```python
from build123d import *

# Parameters (mm, degrees)
MODEL_R             = 1.3
MODEL_R_2           = 1.344067797
MODEL_W             = 12.2
MODEL_H             = 22.8
BOSS_EXTRUDE1_DEPTH = 3


with BuildPart() as part:
    # Model → Boss-Extrude1 (new body)
    with BuildSketch(Plane.XY):
        with BuildLine():
            Line((25.639766947, 69.089607729), (69.59281779, 69.089607729))
            ThreePointArc((69.59281779, 69.089607729), (71.883249375, 68.155605213), (72.834203695, 65.872159696))
            Line((72.834203695, 65.872159696), (72.834203695, 21.872118121))
            ThreePointArc((72.834203695, 21.872118121), (71.882847983, 19.587552286), (69.590964861, 18.653962174))
            Line((69.590964861, 18.653962174), (25.641619876, 18.653962174))
            ThreePointArc((25.641619876, 18.653962174), (23.349724106, 19.587556709), (22.398372881, 21.872138909))
            Line((22.398372881, 21.872138909), (22.398372881, 65.872138909))
            ThreePointArc((22.398372881, 65.872138909), (23.349322718, 68.155600786), (25.639766947, 69.089607729))
        make_face()
        with Locations((25.616288319, 65.871777925)):
            Circle(MODEL_R, mode=Mode.SUBTRACT)
        with Locations((69.616288319, 65.871777925)):
            Circle(MODEL_R, mode=Mode.SUBTRACT)
        with Locations((56.616292368, 43.872138909)):
            Circle(MODEL_R_2, mode=Mode.SUBTRACT)
        with Locations((38.616292368, 43.872138909)):
            Circle(MODEL_R_2, mode=Mode.SUBTRACT)
        with Locations((25.616288319, 21.871777925)):
            Circle(MODEL_R, mode=Mode.SUBTRACT)
        with Locations((69.616288319, 21.871777925)):
            Circle(MODEL_R, mode=Mode.SUBTRACT)
        with Locations((47.616292368, 43.872138909)):
            Rectangle(MODEL_W, MODEL_H, mode=Mode.SUBTRACT)
    extrude(amount=BOSS_EXTRUDE1_DEPTH)


solid = part.part
```
The listing builds one solid part. Answer for the finished solid, in the listing's coordinates (mm). A direction names the side the tool comes from. Give positions to 0.01 mm unless a question says otherwise; leave off trailing zeros. Order: outer loops, then holes, each group sorted by start corner. A loop starts at its lowest first (then second) coordinate and runs counter-clockwise, first axis right, second up.
Item 1: Find the intervals of material crossed by probe 1 along X at (y, z) = (66, 1.3); probe 2 along X at (y, z) = (33, 0.75); probe 3 along Y at (x, z) = (70.5, 1.7), in increasing order.
From the geometry:
probe 1: x = 22.4 to 24.32, 26.91 to 68.32, 70.91 to 72.83
probe 2: x = 22.4 to 41.52, 53.72 to 72.83
probe 3: y = 18.78 to 20.92, 22.83 to 64.92, 66.83 to 68.97
Item 2: The part is cut by section B-B, the plane z = 0.6. Give the vertices of the cut face in (x, y).
From the geometry:
outline: (22.4, 21.87) arc R3.22 ccw to (25.64, 18.65) - (69.59, 18.65) arc R3.22 ccw to (72.83, 21.87) - (72.83, 65.87) arc R3.22 ccw to (69.59, 69.09) - (25.64, 69.09) arc R3.22 ccw to (22.4, 65.87) - close; hole circle Ø2.6 at (25.62, 21.87); hole circle Ø2.6 at (25.62, 65.87); hole circle Ø2.69 at (38.62, 43.87); hole (41.52, 32.47) - (53.72, 32.47) - (53.72, 55.27) - (41.52, 55.27) - close; hole circle Ø2.69 at (56.62, 43.87); hole circle Ø2.6 at (69.62, 21.87); hole circle Ø2.6 at (69.62, 65.87)
Item 3: For a pull along Y with two mould halves and no side action, classify faces 1 (the face through (72.834, 44, 1)), 2 (the face through (53.716, 44, 1)), 3 (the face through (23.324, 68.13, 1.479)) as pulls with the +Y half, pulls with the -Y half, needs draft (parallel to the pull), parting line crosses it, or undercut.
From the geometry:
face 1: needs draft
face 2: undercut
face 3: pulls with the +Y half
Item 4: Which of the six approach directions +Z, -Z, +X, -X, +Y, -Y give full straight-line access (tool end or side, diameter ignored) to faces 4 (the face through (48, 55.272, 1)), 5 (the face through (47.97, 55.43, 0))?
From the geometry:
face 4: +Z, -Z
face 5: -Z, +X, -X, +Y, -Y
Item 5: The part is cut by section A-A, the plane x = 53. Give the vertices of the cut face in (y, z).
From the geometry:
outline: (18.65, 0) - (32.47, 0) - (32.47, 3) - (18.65, 3) - close; (55.27, 0) - (69.09, 0) - (69.09, 3) - (55.27, 3) - close
